from build123d import *

# Parameters (mm, degrees)
BOSS_EXTRUDE1_DEPTH = 12.7
CUT_EXTRUDE1_DEPTH  = 38.486519244
FILLET4_R           = 1.524
FILLET5_R           = 3.81
SKETCH3_R           = 1.27
CUT_EXTRUDE2_DEPTH  = 68.465574925


with BuildPart() as part:
    # Sketch1 → Boss-Extrude1 (new body)
    with BuildSketch(Plane(origin=(0, 0, 0), x_dir=(1, 0, 0), z_dir=(0, 1, 0))):
        Polygon((5.842, 32.385), (-13.97, 32.385), (-13.97, -32.385), (5.842, -32.385), (5.842, -24.765), (-1.27, -24.765), (-1.27, -20.193), (-5.08, -20.193), (-5.08, -12.573), (-1.27, -12.573), (5.842, -12.573), (5.842, 12.573), (-1.27, 12.573), (-5.08, 12.573), (-5.08, 20.193), (-1.27, 20.193), (-1.27, 24.765), (5.842, 24.765), align=None)
    extrude(amount=BOSS_EXTRUDE1_DEPTH)

    # Sketch2 → Cut-Extrude1 (cut, through all)
    with BuildSketch(Plane(origin=(0, 12.7, 0), x_dir=(1, 0, 0), z_dir=(0, 1, 0))):
        Polygon((-1.27, 24.765), (5.842, 26.019037487), (5.842, 24.765), align=None)
        Polygon((-1.27, -24.765), (5.842, -26.019037487), (5.842, -24.765), align=None)
        Polygon((-1.27, -12.573), (5.842, -10.667345343), (5.842, -12.573), align=None)
        Polygon((-1.27, 12.573), (5.842, 10.667345343), (5.842, 12.573), align=None)
    extrude(amount=-CUT_EXTRUDE1_DEPTH, mode=Mode.SUBTRACT)

    # Fillet4
    fillet4_edges = [part.edges().sort_by_distance(p)[0] for p in [
        (-5.08, 6.35, 20.193),
        (-1.27, 6.35, 20.193),
        (-1.27, 6.35, -20.193),
        (-5.08, 6.35, -20.193),
        (-5.08, 6.35, -12.573),
        (-5.08, 6.35, 12.573),
        (-1.27, 6.35, 12.573),
        (-1.27, 6.35, -12.573),
    ]]
    fillet(fillet4_edges, radius=FILLET4_R)

    # Fillet5
    # the kernel refuses this fillet: 3.81 mm, written as the material it takes off along each edge
    with BuildSketch(Plane(origin=(5.842, -9.525, 32.385), x_dir=(-1, 0, 0), z_dir=(0, 1, 0)), Plane(origin=(-13.97, -9.525, 32.385), x_dir=(0, 0, -1), z_dir=(0, 1, 0)), Plane(origin=(-13.97, -9.525, -32.385), x_dir=(1, 0, 0), z_dir=(0, 1, 0)), Plane(origin=(5.842, -9.525, -32.385), x_dir=(0, 0, 1), z_dir=(0, 1, 0))) as fillet5_piece_1:
        with BuildLine():
            CenterArc((FILLET5_R, -FILLET5_R), FILLET5_R, 90, 90)
            Line((0, -FILLET5_R), (0, 0))
            Line((0, 0), (FILLET5_R, 0))
        make_face()
    extrude(amount=31.75, mode=Mode.SUBTRACT)
    with BuildSketch(Plane(origin=(5.842, 20.692423987, -26.019037487), x_dir=(-0.9848077530122095, 0, 0.17364817766692292), z_dir=(0, -1, 0)), Plane(origin=(5.842, 20.692423987, 26.019037487), x_dir=(0, 0, 1), z_dir=(0, -1, 0))) as fillet5_piece_2:
        with BuildLine():
            CenterArc((FILLET5_R * 0.839099631177, FILLET5_R), FILLET5_R, 190, 80)
            Line((-FILLET5_R * 0.145708121835, FILLET5_R * 0.826351822333), (0, 0))
            Line((0, 0), (FILLET5_R * 0.839099631177, 0))
        make_face()
    extrude(amount=28.684847974, mode=Mode.SUBTRACT)
    with BuildSketch(Plane(origin=(5.842, 20.00878956, 10.667345343), x_dir=(0, 0, -1), z_dir=(0, -1, 0)), Plane(origin=(5.842, 20.00878956, -10.667345343), x_dir=(-0.9659258262890701, 0, -0.258819045102514), z_dir=(0, -1, 0))) as fillet5_piece_3:
        with BuildLine():
            CenterArc((FILLET5_R * 0.767326987979, -FILLET5_R), FILLET5_R, 90, 75)
            Line((-FILLET5_R * 0.19859883831, -FILLET5_R * 0.741180954897), (0, 0))
            Line((0, 0), (FILLET5_R * 0.767326987979, 0))
        make_face()
    extrude(amount=27.317579121, mode=Mode.SUBTRACT)

    # Sketch3 → Cut-Extrude2 (cut, through all)
    with BuildSketch(Plane.XY.offset(32.385)):
        with Locations(Location((-9.391956596, 6.35, 0), (0, 0, 127.211471896))):
            Circle(SKETCH3_R)
    extrude(amount=-CUT_EXTRUDE2_DEPTH, mode=Mode.SUBTRACT)


solid = part.part
Input: part model. Units: mm. Frame: model coordinates. A direction names the side the tool comes from. Give positions to 0.01 mm unless a question says otherwise; leave off trailing zeros. Write each loop counter-clockwise with the first axis right and the second up, starting at its lowest first coordinate (ties: lowest second). Pieces come first, ordered by that corner, then holes.
Q1. Pull-direction query (X, two-part tool) for faces 3 (the face through (-4, 6, -32.385)), 4 (the face through (-9.71, 7.58, 0.45)), 5 (the face through (-5.08, 6, 16)); classes: pulls with the +X half, pulls with the -X half, needs draft (parallel to the pull), parting line crosses it, or undercut.
Q2. Material intervals for probe 1 along X at (y, z) = (6.35, -7); probe 2 along Z at (x, y) = (3, 9.5); probe 3 along Z at (x, y) = (-0.5, 3.75) (3 decimals), sorted ascending.
Q3. Set-up query: faces 1 (the face through (-6, 0, 0)), 2 (the face through (-1.27, 6, 23)). Return all of +Z, -Z, +X, -X, +Y, -Y with unobstructed straight access to the full face (end or side cutting, diameter ignored); none if empty.
Q4. Section C-C, the plane z = 9. Output: boundary loops of the cut face in (x, y), plus the area to 3 significant figures.
Q5. First-contact query: P1, Ø0.9, axis at y = 7.5, z = 23.5, coming from the +X side; P2, Ø2.5, axis at y = 6.5, z = -15.5, coming from the +X side. Flat tips, straight axial feed; report the tip coordinate or a pass-through.
Q6. Section B-B, the plane x = 1. Output: boundary loops of the cut face in (y, z) (3 decimals).
Filled in:
1. face 3: needs draft
1. face 4: undercut
1. face 5: pulls with the +X half
2. probe 1: x = -13.97 to -10.66, -8.12 to 5.84
2. probe 2: z = -32.26 to -25.53, -11.43 to 11.43, 25.53 to 32.26
2. probe 3: z = -32.385 to -24.901, -12.367 to 12.367, 24.901 to 32.385
3. face 1: +Z, -Z, +X, -X, -Y
3. face 2: +X, +Y, -Y
4. outline: (-13.97, 0) - (5.63, 0) - (5.63, 12.7) - (-13.97, 12.7) - close; hole circle Ø2.54 at (-9.39, 6.35)
4. area: 244 mm2
5. P1: stops at x = -1.27
5. P2: stops at x = -5.08
6. outline: (0, -32.385) - (12.7, -32.385) - (12.7, -25.165) - (0, -25.165) - close; (0, -11.965) - (12.7, -11.965) - (12.7, 11.965) - (0, 11.965) - close; (0, 25.165) - (12.7, 25.165) - (12.7, 32.385) - (0, 32.385) - close
